Could you check a few things on this model? Use its own coordinates, in mm. Face numbers are marked on the shaded views. A direction names the side the tool comes from. Round coordinates to 2 decimals unless told otherwise and drop trailing zeros. Loops run counter-clockwise (first coordinate to the right, second up) from the corner with the lowest first, then second, coordinate; pieces in that order, holes last. Notation, with made-up numbers: (61, 46.25) -> (108, 46.25) arc R21 ccw to (108, 58.25) -> close; hole circle Ø3 at (-36.75, 24). An arc over 180 degrees is marked (long way). Put each result on its own line as item: value. Start each with the question number.
1. Imagine slicing it at B-B, the plane x = -2.5. Please give me the cut outline in (y, z).
2. Imagine slicing it at C-C, the plane z = -9. Please give me the cut outline in (x, y), and give its area (3 significant figures).
3. Which directions (+Z, -Z, +X, -X, +Y, -Y) give clear straight access to the entire face, cutting with the end or side of a thin tool? Please do the marked faces 4 and 5.
4. I need wall thicknesses on line 1 (Z direction, x = 0.5, y = 4.5); line 2 (Y direction, x = 4, z = -3.5); line 3 (X direction, y = 0.7, z = 0). Which ranges of each line are inside material? Lowest first, please. Write a range as [from, to].
5. Imagine slicing it at A-A, the plane z = 0. Please give me the cut outline in (x, y), and give its area (3 significant figures).
6. Imagine slicing it at D-D, the plane x = 4.75. Please give me the cut outline in (y, z), and give its area (3 significant figures).
7. If we mould it in two halves opening along Y, with no side actions, what happens to the marked faces 1, 2 and 3? For each: pulls with the +Y half, pulls with the -Y half, needs draft (parallel to the pull), parting line crosses it, or undercut.
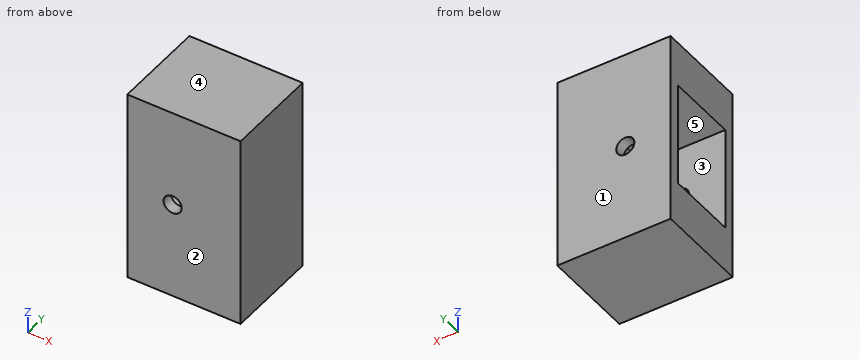
```python
from build123d import *

# Parameters (mm, degrees)
SKETCH1_W           = 25
SKETCH1_H           = 43
BOSS_EXTRUDE1_DEPTH = 20.67
SKETCH2_W           = 23
SKETCH2_H           = 15.735859414
CUT_EXTRUDE1_DEPTH  = 18
SKETCH3_R           = 2
CUT_EXTRUDE2_DEPTH  = 33.338041066


with BuildPart() as part:
    # Sketch1 → Boss-Extrude1 (new body)
    with BuildSketch(Plane(origin=(0, 0, 0), x_dir=(1, 0, 0), z_dir=(0, 1, 0))):
        Rectangle(SKETCH1_W, SKETCH1_H)
    extrude(amount=BOSS_EXTRUDE1_DEPTH)

    # Sketch2 → Cut-Extrude1 (cut)
    with BuildSketch(Plane.ZY.offset(12.5)):
        with Locations((0, 10.335)):
            Rectangle(SKETCH2_W, SKETCH2_H)
    extrude(amount=-CUT_EXTRUDE1_DEPTH, mode=Mode.SUBTRACT)

    # Sketch3 → Cut-Extrude2 (cut, through all)
    with BuildSketch(Plane.XZ):
        with Locations(Location((-2.5, 0, 0), (0, 0, 270))):
            Circle(SKETCH3_R)
    extrude(amount=-CUT_EXTRUDE2_DEPTH, mode=Mode.SUBTRACT)


solid = part.part
```
Entries:
1. outline: (0, -21.5) -> (20.67, -21.5) -> (20.67, -2) -> (18.2, -2) -> (18.2, -11.5) -> (2.47, -11.5) -> (2.47, -2) -> (0, -2) -> close; (0, 2) -> (2.47, 2) -> (2.47, 11.5) -> (18.2, 11.5) -> (18.2, 2) -> (20.67, 2) -> (20.67, 21.5) -> (0, 21.5) -> close
2. outline: (-12.5, 0) -> (12.5, 0) -> (12.5, 20.67) -> (-12.5, 20.67) -> (-12.5, 18.2) -> (5.5, 18.2) -> (5.5, 2.47) -> (-12.5, 2.47) -> close
2. area: 234 mm^2
3. face 4: +Z, +X, -X, +Y, -Y
3. face 5: -X
4. line 1: [-21.5, -11.5], [11.5, 21.5]
4. line 2: [0, 2.47], [18.2, 20.67]
4. line 3: [-12.5, -4.5], [-0.5, 12.5]
5. outline: (-12.5, 0) -> (-4.5, 0) -> (-4.5, 2.47) -> (-12.5, 2.47) -> close; (-12.5, 18.2) -> (-4.5, 18.2) -> (-4.5, 20.67) -> (-12.5, 20.67) -> close; (-0.5, 0) -> (12.5, 0) -> (12.5, 20.67) -> (-0.5, 20.67) -> (-0.5, 18.2) -> (5.5, 18.2) -> (5.5, 2.47) -> (-0.5, 2.47) -> close
5. area: 214 mm^2
6. outline: (0, -21.5) -> (20.67, -21.5) -> (20.67, 21.5) -> (0, 21.5) -> close; hole (2.47, -11.5) -> (18.2, -11.5) -> (18.2, 11.5) -> (2.47, 11.5) -> close
6. area: 527 mm^2
7. face 1: pulls with the +Y half
7. face 2: pulls with the -Y half
7. face 3: undercut
